Input: part model. Units: mm. Frame: model coordinates. A direction names the side the tool comes from. Round coordinates to 2 decimals unless told otherwise and drop trailing zeros. Loops run counter-clockwise (first coordinate to the right, second up) from the corner with the lowest first, then second, coordinate; pieces in that order, holes last. Notation, with made-up numbers: M 32,-11 L 49,-11 A17 ccw 49,12 Z; hole C -38,50 d2. An arc over 180 degrees is marked long. Return JSON: item names as keys, results as strings. Group by question number.
1) Mould query, pull axis X, two halves, no side actions, for faces 1 (the face through (-33, 0, 30)), 2 (the face through (-38.75, -3.11, 13.47)), 3 (the face through (-41.394, -2, 42)). Classes: +X half, -X half, draft (parallel to the pull), parting line (faces both ways), or undercut.
2) Access query for faces 4 (the face through (-33, -2, 4.571)), 5 (the face through (-38.75, -0.44, 13.47)), 6 (the face through (-22.344, -2, 32)). Directions: +Z, -Z, +X, -X, +Y, -Y. A direction counts if a zero-diameter tool reaches every point of the face in a straight line with its end or side. Return the directions, or none.
3) Section C-C (z = 44.5). Output: boundary loops of the cut face in (x, y), plus the area to 3 significant figures.
4) Section A-A (y = -2.1). Output: boundary loops of the cut face in (x, z), plus the area to 3 significant figures.
5) Contact query for flat-ended pins moving along their axis: P1, Ø1.4, axis at x = -36, y = -2, coming from the +Z side; P2, Ø1.5, axis at y = -3, z = 41.5, coming from the -X side. Output: stop coordinate, or through.
6) Section B-B (x = -33). Output: boundary loops of the cut face in (y, z).
7) Material intervals for line 1 (Y direction, x = -29.25, z = 15); line 2 (Z direction, x = -36, y = -2.3); line 3 (X direction, y = -0.95, z = 23), sorted ascending. Write a range as from..to.
8) Section D-D (x = -42.25). Output: boundary loops of the cut face in (y, z).
from build123d import *

# Parameters (mm, degrees)
F0_R     = 1.27
F1_DEPTH = 3.556
F2_W     = 19.05
F2_H     = 1.778
F3_DEPTH = 48.26


with BuildPart() as f1:
    # F0 (on Front) → F1 (new body)
    with BuildSketch(Plane.XZ):
        Polygon((-21.582347, 55.370963), (-43.807347, 55.370963), (-40.730689, 21.41812), (-36.822347, 16.094806), (-40.730689, 10.771491), (-43.807347, 4.570963), (-21.582347, 4.570963), align=None)
        with Locations((-37.126201, 50.380394)):
            Circle(F0_R, mode=Mode.SUBTRACT)
        with Locations((-26.401985, 50.352663)):
            Circle(F0_R, mode=Mode.SUBTRACT)
    extrude(amount=F1_DEPTH)

    # F2 (on face) → F3 (cut)
    with BuildSketch(Plane.XY.offset(55.370963)):
        with Locations((-31.869347, -1.778)):
            Rectangle(F2_W, F2_H)
    extrude(amount=-F3_DEPTH, mode=Mode.SUBTRACT)


solid = f1.part
Returned:
{
 "1": {"face 1": "draft", "face 2": "-X half", "face 3": "undercut"},
 "2": {"face 4": "-Z, +X, -X, +Y, -Y", "face 5": "-X, +Y, -Y", "face 6": "+Z"},
 "3": {"outline": "M -42.82,-3.56 L -21.58,-3.56 L -21.58,0 L -42.82,0 Z; hole M -41.39,-2.67 L -22.34,-2.67 L -22.34,-0.89 L -41.39,-0.89 Z", "area": "41.7 mm^2"},
 "4": {"outline": "M -43.81,4.57 L -21.58,4.57 L -21.58,55.37 L -22.34,55.37 L -22.34,7.11 L -41.39,7.11 L -41.39,9.43 Z; M -43.81,55.37 L -41.39,28.74 L -41.39,55.37 Z", "area": "125 mm^2"},
 "5": {"P1": "stops at z = 55.37", "P2": "stops at x = -42.62"},
 "6": {"outline": "M -3.56,4.57 L 0,4.57 L 0,55.37 L -0.89,55.37 L -0.89,7.11 L -2.67,7.11 L -2.67,55.37 L -3.56,55.37 Z"},
 "7": {"line 1": "y = -3.56..-2.67, -0.89..0", "line 2": "z = 4.57..7.11", "line 3": "x = -22.34..-21.58"},
 "8": {"outline": "M -3.56,4.57 L 0,4.57 L 0,7.71 L -3.56,7.71 Z; M -3.56,38.18 L 0,38.18 L 0,55.37 L -3.56,55.37 Z"}
}
